CAD build for the part. Positions are in the model's coordinates, mm. A direction names the side the tool comes from. Coordinates: 2 decimals unless noted, no trailing zeros. Order: outer loops, then holes, each group sorted by start corner. A loop starts at its lowest first (then second) coordinate and runs counter-clockwise, first axis right, second up.
from build123d import *

# Parameters (mm, degrees)
F1_DEPTH = 31.75
F3_D     = 5.08
F5_D     = 5.08


with BuildPart() as f1:
    # F0 (on Top) → F1 (new body)
    with BuildSketch(Plane.XY):
        Polygon((-81.060801, -28.900409), (-81.060801, 47.299591), (103.089199, 47.299591), (103.089199, -28.900409), (141.189199, -28.900409), (141.189199, -23.820409), (108.169199, -23.820409), (108.169199, 52.379591), (-86.140801, 52.379591), (-86.140801, -23.820409), (-119.160801, -23.820409), (-119.160801, -28.900409), align=None)
    extrude(amount=F1_DEPTH)

    # F3 (through all)
    with Locations(Plane(origin=(0, -23.820409, 0), x_dir=(-1, 0, 0), z_dir=(0, 1, 0))):
        with Locations((102.650801, 15.875)):
            Hole(F3_D / 2)

    # F5 (through all)
    with Locations(Plane(origin=(0, -23.820409, 0), x_dir=(-1, 0, 0), z_dir=(0, 1, 0))):
        with Locations((-124.679199, 15.875)):
            Hole(F5_D / 2)


solid = f1.part
1) Slice it at C-C (x = -45). List the corners of the cut face in (y, z), plus the area to 3 significant figures.
2) Pin check, flat tips, straight feed: P1, Ø16, axis at x = -106, z = 22, coming from the +Y side; P2, Ø16, axis at y = 17, z = 23.5, coming from the -X side; P3, Ø12, axis at x = 14.5, z = 22, coming from the -Y side; P4, Ø10, axis at x = -77, z = 15, coming from the -Y side. Stop position of each tip, or through.
3) Drill centre lines: probe 1 along X at (y, z) = (44.5, 26.5); probe 2 along Y at (x, z) = (-24, 6); probe 3 along Y at (x, z) = (-88, 23). Where is each one in solid material? Low to high.
4) Which spindle directions (+Z, -Z, +X, -X, +Y, -Y) get a long thin tool onto all of the face, cutting with end or side? Do faces 1 (the flat face through (141.189, -26, 16)), 2 (the flat face through (10, 47.3, 16)), 3 (the flat face through (108.169, 14, 16)), 4 (the flat face through (-102, -23.82, 12)). Say none if no direction does.
5) Slice it at B-B (z = 22.5). List the corners of the cut face in (x, y).
6) Two-plate mould, pull along Z, no slides. Class faces 5 (the cylindrical face through (124.1, -26.4, 13.4)), 6 (the flat face through (121.9, -28.9, 15.7)), 7 (the flat face through (1, 48, 31.75)): released by +Z, released by -Z, zero draft, split by the parting line, or undercut.
7) Slice it at A-A (y = 39). List the corners of the cut face in (x, z), plus the area to 3 significant figures.
Worked out:
1. outline: (47.3, 0) - (52.38, 0) - (52.38, 31.75) - (47.3, 31.75) - close
1. area: 161 mm2
2. P1: stops at y = -23.82
2. P2: stops at x = -86.14
2. P3: stops at y = 47.3
2. P4: stops at y = -28.9
3. probe 1: x = -86.14 to -81.06, 103.09 to 108.17
3. probe 2: y = 47.3 to 52.38
3. probe 3: y = -28.9 to -23.82
4. face 1: +Z, -Z, +X, +Y, -Y
4. face 2: +Z, -Z, -Y
4. face 3: +Z, -Z, +X, +Y
4. face 4: +Z, -Z, -X, +Y
5. outline: (-119.16, -28.9) - (-81.06, -28.9) - (-81.06, 47.3) - (103.09, 47.3) - (103.09, -28.9) - (141.19, -28.9) - (141.19, -23.82) - (108.17, -23.82) - (108.17, 52.38) - (-86.14, 52.38) - (-86.14, -23.82) - (-119.16, -23.82) - close
6. face 5: undercut
6. face 6: zero draft
6. face 7: released by +Z
7. outline: (-86.14, 0) - (-81.06, 0) - (-81.06, 31.75) - (-86.14, 31.75) - close; (103.09, 0) - (108.17, 0) - (108.17, 31.75) - (103.09, 31.75) - close
7. area: 323 mm2
